```python
from build123d import *

# Parameters (mm, degrees)
CROQUIS1_W              = 72
CROQUIS1_H              = 67
SALIENTE_EXTRUIR1_DEPTH = 3
CROQUIS3_R              = 1.625
CROQUIS3_R_2            = 1.5
CROQUIS3_RX             = 3
CROQUIS3_RY             = 2
CORTAR_EXTRUIR1_DEPTH   = 3


with BuildPart() as part:
    # Croquis1 → Saliente-Extruir1 (new body)
    with BuildSketch(Plane.XY):
        with Locations((122.25, -8.443705264)):
            Rectangle(CROQUIS1_W, CROQUIS1_H)
    extrude(amount=SALIENTE_EXTRUIR1_DEPTH)

    # Croquis3 → Cortar-Extruir1 (cut)
    with BuildSketch(Plane(origin=(0, 0, 0), x_dir=(-1, 0, 0), z_dir=(0, 0, -1))):
        with Locations((-122.25, -35.943705264)):
            Circle(CROQUIS3_R)
        with Locations((-97.25, 22.056294736)):
            Circle(CROQUIS3_R)
        with Locations((-137.977922061, 8.284216797)):
            Circle(CROQUIS3_R_2)
        with Locations((-129.908742812, 12.942959609)):
            Circle(CROQUIS3_R_2)
        with Locations((-134.25, 11.144752004)):
            Circle(CROQUIS3_R_2)
        with Locations((-128.744057109, 8.596293391)):
            Circle(CROQUIS3_R_2)
        with Locations((-125.25, 13.556294736)):
            Circle(CROQUIS3_R_2)
        with Locations((-120.591257188, 12.942959609)):
            Circle(CROQUIS3_R_2)
        with Locations((-121.755942891, 8.596293391)):
            Circle(CROQUIS3_R_2)
        with Locations((-116.25, 11.144752004)):
            Circle(CROQUIS3_R_2)
        with Locations((-112.522077939, 8.284216797)):
            Circle(CROQUIS3_R_2)
        with Locations((-115.704058454, 5.102236282)):
            Circle(CROQUIS3_R_2)
        with Locations((-109.661542732, 4.556294736)):
            Circle(CROQUIS3_R_2)
        with Locations((-107.25, -4.443705264)):
            Circle(CROQUIS3_R_2)
        with Locations((-107.863335127, 0.215037548)):
            Circle(CROQUIS3_R_2)
        with Locations((-112.210001345, -0.949648155)):
            Circle(CROQUIS3_R_2)
        with Locations((-116.556667563, -2.114333858)):
            Circle(CROQUIS3_R_2)
        with Locations((-118.886038969, 1.920255767)):
            Circle(CROQUIS3_R_2)
        with Locations((-122.068019485, -1.261724749)):
            Circle(CROQUIS3_R_2)
        with Locations((-122.920628594, 4.249627173)):
            Circle(CROQUIS3_R_2)
        with Locations((-127.579371406, 4.249627173)):
            Circle(CROQUIS3_R_2)
        with Locations((-131.613961031, 1.920255767)):
            Circle(CROQUIS3_R_2)
        with Locations((-128.431980515, -1.261724749)):
            Circle(CROQUIS3_R_2)
        with Locations((-134.795941546, 5.102236282)):
            Circle(CROQUIS3_R_2)
        with Locations((-140.838457268, 4.556294736)):
            Circle(CROQUIS3_R_2)
        with Locations((-143.25, -4.443705264)):
            Circle(CROQUIS3_R_2)
        with Locations((-142.636664873, 0.215037548)):
            Circle(CROQUIS3_R_2)
        with Locations((-138.289998655, -0.949648155)):
            Circle(CROQUIS3_R_2)
        with Locations((-133.943332437, -2.114333858)):
            Circle(CROQUIS3_R_2)
        with Locations((-133.943332437, -6.77307667)):
            Circle(CROQUIS3_R_2)
        with Locations((-125.25, -4.443705264)):
            Circle(CROQUIS3_R_2)
        with Locations((-128.431980515, -7.625685779)):
            Circle(CROQUIS3_R_2)
        with Locations((-122.068019485, -7.625685779)):
            Circle(CROQUIS3_R_2)
        with Locations((-116.556667563, -6.77307667)):
            Circle(CROQUIS3_R_2)
        with Locations((-107.863335127, -9.102448076)):
            Circle(CROQUIS3_R_2)
        with Locations((-112.210001345, -7.937762373)):
            Circle(CROQUIS3_R_2)
        with Locations((-109.661542732, -13.443705264)):
            Circle(CROQUIS3_R_2)
        with Locations((-112.522077939, -17.171627325)):
            Circle(CROQUIS3_R_2)
        with Locations((-118.886038969, -10.807666295)):
            Circle(CROQUIS3_R_2)
        with Locations((-127.579371406, -13.137037701)):
            Circle(CROQUIS3_R_2)
        with Locations((-122.920628594, -13.137037701)):
            Circle(CROQUIS3_R_2)
        with Locations((-115.704058454, -13.98964681)):
            Circle(CROQUIS3_R_2)
        with Locations((-121.755942891, -17.483703919)):
            Circle(CROQUIS3_R_2)
        with Locations((-116.25, -20.032162532)):
            Circle(CROQUIS3_R_2)
        with Locations((-120.591257188, -21.830370137)):
            Circle(CROQUIS3_R_2)
        with Locations((-125.25, -22.443705264)):
            Circle(CROQUIS3_R_2)
        with Locations((-128.744057109, -17.483703919)):
            Circle(CROQUIS3_R_2)
        with Locations((-131.613961031, -10.807666295)):
            Circle(CROQUIS3_R_2)
        with Locations((-134.795941546, -13.98964681)):
            Circle(CROQUIS3_R_2)
        with Locations((-138.289998655, -7.937762373)):
            Circle(CROQUIS3_R_2)
        with Locations((-142.636664873, -9.102448076)):
            Circle(CROQUIS3_R_2)
        with Locations((-140.838457268, -13.443705264)):
            Circle(CROQUIS3_R_2)
        with Locations((-137.977922061, -17.171627325)):
            Circle(CROQUIS3_R_2)
        with Locations((-134.25, -20.032162532)):
            Circle(CROQUIS3_R_2)
        with Locations((-129.908742812, -21.830370137)):
            Circle(CROQUIS3_R_2)
        with Locations(Location((-145.464659991, 17.041580897), (0, 0, -46.745301972))):
            Ellipse(CROQUIS3_RX, CROQUIS3_RY)
        with Locations(Location((-105.035340009, -25.928991425), (0, 0, -46.745301972))):
            Ellipse(CROQUIS3_RX, CROQUIS3_RY)
    extrude(amount=-CORTAR_EXTRUIR1_DEPTH, mode=Mode.SUBTRACT)


solid = part.part
```
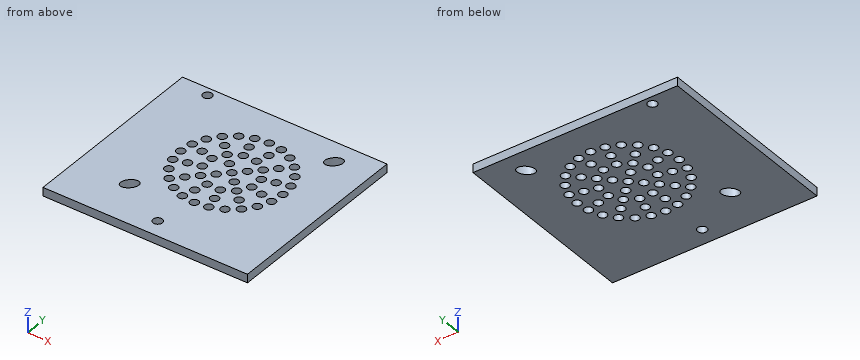
Work out the finished part from the listing and answer in its coordinate system (mm). Give positions to 0.01 mm unless a question says otherwise; leave off trailing zeros. Write each loop counter-clockwise with the first axis right and the second up, starting at its lowest first coordinate (ties: lowest second). Pieces come first, ordered by that corner, then holes.
(1) Straight lines are drawn through the part: line 1 (X direction, y = 13, z = 1.25); line 2 (Y direction, x = 120, z = 2.7); line 3 (X direction, y = 14, z = 0.8). For each, find the intervals that lie inside material, in ascending order.
Final values:
line 1: x = 86.25 to 119.09, 122.09 to 123.86, 126.64 to 128.41, 131.41 to 158.25
line 2: y = -41.94 to -23.21, -20.45 to -11.81, -9.8 to 0.92, 2.92 to 11.56, 14.32 to 25.06
line 3: x = 86.25 to 119.53, 121.66 to 123.82, 126.68 to 128.84, 130.97 to 158.25
(2) The part is cut by section B-B on z = 1.6. Count the separate pieces of the cut face and the enclosed holes in it, plus the area to 3 significant figures.
Final values:
separate pieces: 1
enclosed holes: 57
area: 4,400 mm2
(3) The part is cut by section A-A on x = 134.25. Write down the section's boundary in (y, z).
Final values:
outline: (-41.94, 0) - (-21.53, 0) - (-21.53, 3) - (-41.94, 3) - close; (-18.53, 0) - (-15.39, 0) - (-15.39, 3) - (-18.53, 3) - close; (-12.59, 0) - (-8.24, 0) - (-8.24, 3) - (-12.59, 3) - close; (-5.3, 0) - (-3.58, 0) - (-3.58, 3) - (-5.3, 3) - close; (-0.65, 0) - (3.71, 0) - (3.71, 3) - (-0.65, 3) - close; (6.5, 0) - (9.64, 0) - (9.64, 3) - (6.5, 3) - close; (12.64, 0) - (25.06, 0) - (25.06, 3) - (12.64, 3) - close
